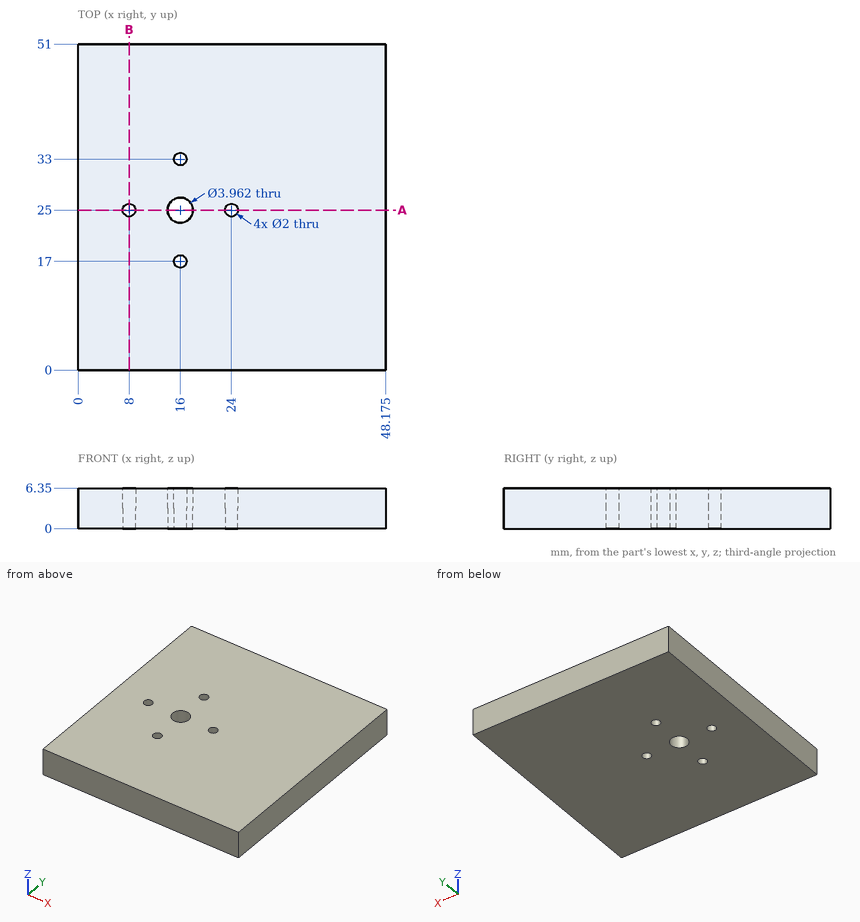
The drawing under review shows one solid part. Ordinate dimensions are in mm from its lowest x, y, z. Round coordinates to 2 decimals unless told otherwise and drop trailing zeros. Loops run counter-clockwise (first coordinate to the right, second up) from the corner with the lowest first, then second, coordinate; pieces in that order, holes last. Notation, with made-up numbers: (65, 44.25) - (118, 44.25) arc R19 cw to (118, 73.25) - close; hole circle Ø8 at (-12, -33). An arc over 180 degrees is marked (long way). One line per item, written item: value. Start each with the question number.
1) To check wall thickness, follow L1, parallel to X at y = 25, z = 2.3 (1 decimal); L2, parallel to Y at x = 16, z = 2; L3, parallel to X at y = 17, z = 4.1 (1 decimal). State the ranges of each line that lie inside material, in increasing order. Write a range as from..to.
2) Consider section A-A on y = 25. Give the number of separate pieces and of enclosed holes in the cut face, then the cut area to 3 significant figures.
3) Consider section B-B on x = 8. Give the boundary of the cut face in (y, z).
Reported:
1. L1: x = 0..7, 9..14, 18..23, 25..48.2
1. L2: y = 0..16, 18..23.02, 26.98..32, 34..51
1. L3: x = 0..15, 17..48.2
2. separate pieces: 4
2. enclosed holes: 0
2. area: 255 mm^2
3. outline: (0, 0) - (24, 0) - (24, 6.35) - (0, 6.35) - close; (26, 0) - (51, 0) - (51, 6.35) - (26, 6.35) - close
